Autodesk Inventor part; units mm, degrees
ref_plane "YZ Plane" through (0, 0, 0) normal (1, 0, 0) x (0, 1, 0)
ref_plane "XZ Plane" through (0, 0, 0) normal (0, 1, 0) x (-1, 0, 0)
ref_plane "XY Plane" through (0, 0, 0) normal (0, 0, 1) x (1, 0, 0)
sketch "Sketch1" plane through (0, 0, 0) normal (0, 1, 0) x (-1, 0, 0)
  line L0 (0, 0) -> (0, -14)
  circle A0 centre (0, -7) radius 8.25
  circle A1 centre (0, -7) radius 10.5
  dimension "d0" = 14
  dimension "d1" = 16.5
  dimension "d2" = 21
extrude "Extrusion1" add sketch "Sketch1" along normal blind 6
sketch "Sketch2" plane through (0, 6, -7) normal (0, 1, 0) x (1, 0, 0)
  line L0 (10.5, -10.5) -> (-10.5, -10.5)
  line L1 (-10.5, -10.5) -> (-10.5, 10.5)
  line L2 (-10.5, 10.5) -> (10.5, 10.5)
  line L3 (10.5, 10.5) -> (10.5, -10.5)
  line L4 (10.5, -10.5) -> (-10.5, 10.5) construction
  line L5 (-10.5, -10.5) -> (10.5, 10.5) construction
  circle A0 centre (0, 0) radius 10.5
  point P0 (0, -7)
extrude "Extrusion2" add sketch "Sketch2" against normal blind 6 contours L0 A0 L3 | L0 L1 A0 | A0 L2 L3 | L1 L2 A0
sketch "Sketch4" plane through (0, 6, 0) normal (0, 1, 0) x (1, 0, 0)
  circle A0 centre (0, 7) radius 8.25
  line L0 (0, 7) -> (0, -0.25)
  line L1 (0, -0.25) -> (-3.937, -0.25)
  line L2 (3.937, -0.25) -> (-3.937, -0.25)
  point P0 (0, 0)
  dimension "d14" = 7.25
extrude "Extrusion4" add sketch "Sketch4" against normal blind 6 contours L1 L2 A0 picked at (1.9893, -0.4987)
pattern_circular "Circular Pattern2" count 6 over 360 about axis through (0, 0, -7) along (0, 1, 0) of "Extrusion4"
sketch "Sketch5" plane through (0, 6, 0) normal (0, 1, 0) x (1, 0, 0)
  line L0 (-4.3102, -0.0345) -> (-8.2472, 6.7845)
  line L1 (-6.2787, 3.375) -> (6.2787, 10.625)
  line L2 (4.3102, 14.0345) -> (8.2472, 7.2155)
  line L3 (8.2472, 6.7845) -> (4.3102, -0.0345)
  line L4 (6.2787, 3.375) -> (-6.2787, 10.625)
  line L5 (-4.3102, 14.0345) -> (-8.2472, 7.2155)
  line L6 (3.937, 14.25) -> (-3.937, 14.25)
  line L7 (0, 14.25) -> (0, -0.25)
  line L8 (3.937, -0.25) -> (-3.937, -0.25)
  circle A0 centre (0, 7) radius 9.625
  line L9 (12.5, 19.5) -> (-12.5, 19.5)
  line L10 (-12.5, 19.5) -> (-12.5, -5.5)
  line L11 (-12.5, -5.5) -> (12.5, -5.5)
  line L12 (12.5, -5.5) -> (12.5, 19.5)
  line L13 (12.5, 19.5) -> (-12.5, -5.5) construction
  line L14 (-12.5, 19.5) -> (12.5, -5.5) construction
  point P0 (0, 0)
  dimension "d20" = 19.25
  dimension "d21" = 25
  dimension "d22" = 25
extrude "Extrusion5" add sketch "Sketch5" along normal blind 20
sketch "Sketch6" plane through (0, 6, 0) normal (0, -1, 0) x (1, 0, 0)
  line L0 (-10.5, -17.5) -> (10.5, -17.5)
  line L1 (10.5, -17.5) -> (10.5, 3.5)
  line L2 (10.5, 3.5) -> (-10.5, 3.5)
  line L3 (-10.5, 3.5) -> (-10.5, -17.5)
  circle A0 centre (0, -7) radius 9.625
  line L4 (-10.5, -17.5) -> (10.5, 3.5) construction
  line L5 (10.5, -17.5) -> (-10.5, 3.5) construction
  line L6 (-12.5, -19.5) -> (12.5, -19.5)
  line L7 (12.5, -19.5) -> (12.5, 5.5)
  line L8 (12.5, 5.5) -> (-12.5, 5.5)
  line L9 (-12.5, 5.5) -> (-12.5, -19.5)
  line L10 (-12.5, -19.5) -> (12.5, 5.5) construction
  line L11 (12.5, -19.5) -> (-12.5, 5.5) construction
  point P0 (0, 0)
extrude "Extrusion6" add sketch "Sketch6" along normal blind 6 contours L9 L8 L7 L6
sketch "Sketch8" plane through (-12.5, 26, 5.5) normal (0, 0, 1) x (1, 0, 0)
  line L0 (0, 0) -> (25, 0)
  line L1 (0, 0) -> (-17.5, 0)
  line L2 (25, 0) -> (42.5, 0)
  line L3 (0, 0) -> (-17.5, 0)
  line L4 (-17.5, 0) -> (-17.5, -26)
  line L5 (-17.5, -26) -> (0, -26)
  line L6 (0, -26) -> (0, 0)
  line L7 (25, 0) -> (42.5, 0)
  line L8 (42.5, 0) -> (42.5, -26)
  line L9 (42.5, -26) -> (25, -26)
  line L10 (25, -26) -> (25, 0)
  point P0 (12.5, -26)
  dimension "d27" = 17.5
  dimension "d28" = 17.5
extrude "Extrusion7" add sketch "Sketch8" against normal blind 25
sketch "Sketch9" plane through (-30, 0, 5.5) normal (0, 0, 1) x (1, 0, 0)
  line L0 (0, 26) -> (-15, 26)
  line L1 (-15, 26) -> (-15, 0)
  line L2 (-15, 0) -> (0, 0)
  line L3 (0, 0) -> (0, 26)
  line L4 (60, 26) -> (75, 26)
  line L5 (75, 26) -> (75, 0)
  line L6 (75, 0) -> (60, 0)
  line L7 (60, 0) -> (60, 26)
  point P0 (30, 0)
  dimension "d31" = 15
  dimension "d32" = 15
extrude "Extrusion8" add sketch "Sketch9" against normal blind 61.25
sketch "Sketch10" plane through (-45, 0, 5.5) normal (-1, 0, 0) x (0, 0, 1)
  line L0 (-61.25, 0) -> (-61.25, 26)
  line L1 (-61.25, 13) -> (-35, 13)
  circle A0 centre (-48.125, 13) radius 4.125
  point P0 (-5.5, 0)
  dimension "d35" = 26.25
  dimension "d36" = 8.25
extrude "Extrusion9" cut sketch "Sketch10" against normal through all
sketch "Sketch11" plane through (0, 26, 0) normal (0, 1, 0) x (1, 0, 0)
  line L0 (30, 19.5) -> (30, 24.5)
  line L1 (30, 19.5) -> (30, 55.75)
  line L2 (30, 19.5) -> (25, 19.5)
  line L3 (25, 19.5) -> (30, 24.5)
  line L4 (-30, 19.5) -> (-30, 24.5)
  line L5 (-30, 19.5) -> (-30, 55.75)
  line L6 (-30, 19.5) -> (-25, 19.5)
  line L7 (30, 19.5) -> (-30, 19.5)
  line L8 (-25, 19.5) -> (-30, 24.5)
  point P0 (0, 0)
  dimension "d39" = 5
  dimension "d40" = 5
  dimension "d41" = 5
  dimension "d42" = 5
extrude "Extrusion10" add sketch "Sketch11" against normal blind 26
sketch "Sketch12" plane through (0, 26, 0) normal (0, 1, 0) x (1, 0, 0)
  line L0 (-45, -5.5) -> (-45, 55.75)
  line L1 (45, -5.5) -> (-45, -5.5)
  line L2 (-45, -5.5) -> (-45, 24.5)
  line L3 (-45, 24.5) -> (45, 24.5)
  line L4 (45, 24.5) -> (45, -5.5)
  point P0 (0, 0)
properties part number "FretterMount"
Could you check a few things on this model? Use its own coordinates, in mm. A direction names the side the tool comes from. Give positions to 0.01 mm unless a question says otherwise; leave off trailing zeros. Order: outer loops, then holes, each group sorted by start corner. A loop starts at its lowest first (then second) coordinate and runs counter-clockwise, first axis right, second up.
1. For pin 1 (3 mm diameter, centred on x = 0, y = 2, fed in from -Z), with a flat end and sliding along its axis, tell me the tip position at first contact or that it passes through.
Answers below:
pin 1: stops at z = -19.5
2. Suppose I cut it at C-C (x = 0). Write out the boundary of the cut face in (y, z) (3 decimals).
Answers below:
outline: (0, -19.5) - (26, -19.5) - (26, -16.625) - (6, -16.625) - (6, -14.25) - (0, -14.25) - close; (0, 0.25) - (6, 0.25) - (6, 2.625) - (26, 2.625) - (26, 5.5) - (0, 5.5) - close
3. Suppose I cut it at D-D (y = 20.5). Write out the boundary of the cut face in (x, z) (3 decimals), plus the area to 3 significant figures.
Answers below:
outline: (-45, -55.75) - (-30, -55.75) - (-30, -24.5) - (-25, -19.5) - (25, -19.5) - (30, -24.5) - (30, -55.75) - (45, -55.75) - (45, 5.5) - (-45, 5.5) - close; hole circle Ø19.25 at (0, -7)
area: 3,070 mm2
4. Which directions (+Z, -Z, +X, -X, +Y, -Y) give clear straight access to the entire face, cutting with the end or side of a thin tool? Please do faces 1 (the flat face through (6, 6, -12)), 2 (the flat face through (0, 13, -19.5)), 3 (the flat face through (-1, 26, -19)), 4 (the flat face through (6.306, 3.042, -3.423)).
Answers below:
face 1: +Y
face 2: -Z, +Y, -Y
face 3: +Z, -Z, +X, -X, +Y
face 4: +Y, -Y
5. Suppose I cut it at B-B (z = -37). Write out the boundary of the cut face in (x, y).
Answers below:
outline: (-45, 0) - (-30, 0) - (-30, 26) - (-45, 26) - close; (30, 0) - (45, 0) - (45, 26) - (30, 26) - close
6. Thinking about a two-plate mould opening in Z: for faces 5 (the flat face through (-6.306, 3.042, -10.577)), 6 (the flat face through (-30, 13, -36)), 7 (the flat face through (-27.5, 13.2, -22)), 8 (the flat face through (0, 3, 0.25)), which applies, +Z half, -Z half, draft (parallel to the pull), parting line (faces both ways), or undercut?
Answers below:
face 5: undercut
face 6: draft
face 7: -Z half
face 8: undercut
7. I need wall thicknesses on L1, parallel to Z at x = -37.5, y = 13; L2, parallel to X at y = 24.25, z = -31; L3, parallel to X at y = 14.75, z = -7 (3 decimals). Which ranges of each line are inside material? Lowest first, please.
Answers below:
L1: z = -55.75 to -46.75, -38.5 to 5.5
L2: x = -45 to -30, 30 to 45
L3: x = -45 to -9.625, 9.625 to 45
8. Suppose I cut it at A-A (y = 13). Write out the boundary of the cut face in (x, z) (3 decimals), plus the area to 3 significant figures.
Answers below:
outline: (-45, -55.75) - (-30, -55.75) - (-30, -46.75) - (-45, -46.75) - close; (-45, -38.5) - (-30, -38.5) - (-30, -24.5) - (-25, -19.5) - (25, -19.5) - (30, -24.5) - (30, -38.5) - (45, -38.5) - (45, 5.5) - (-45, 5.5) - close; (30, -55.75) - (45, -55.75) - (45, -46.75) - (30, -46.75) - close; hole circle Ø19.25 at (0, -7)
area: 2,820 mm2
